```python
from build123d import *

# Parameters (mm, degrees)
SKETCH1_R           = 6.625
BOSS_EXTRUDE1_DEPTH = 3
SKETCH2_R           = 7.6
CUT_EXTRUDE1_DEPTH  = 2
BOSS_EXTRUDE2_DEPTH = 90


with BuildPart() as part:
    # Sketch1 → Boss-Extrude1 (new body)
    with BuildSketch(Plane(origin=(0, 0, 0), x_dir=(1, 0, 0), z_dir=(0, 1, 0))):
        with BuildLine():
            Line((58, -58), (58, 58))
            ThreePointArc((58, 58), (0, 116), (-58, 58))
            Line((-58, 58), (-58, -58))
            ThreePointArc((-58, -58), (0, -116), (58, -58))
        make_face()
        with Locations((0, 106.699495206)):
            Circle(SKETCH1_R, mode=Mode.SUBTRACT)
        with Locations((42.175, 33.650252397)):
            Circle(SKETCH1_R, mode=Mode.SUBTRACT)
        with Locations((-42.175, 33.650252397)):
            Circle(SKETCH1_R, mode=Mode.SUBTRACT)
        with Locations((-42.175, -33.650252397)):
            Circle(SKETCH1_R, mode=Mode.SUBTRACT)
        with Locations((0, -106.699495206)):
            Circle(SKETCH1_R, mode=Mode.SUBTRACT)
        with Locations((42.175, -33.650252397)):
            Circle(SKETCH1_R, mode=Mode.SUBTRACT)
    extrude(amount=BOSS_EXTRUDE1_DEPTH)

    # Sketch2 → Cut-Extrude1 (cut)
    with BuildSketch(Plane.XZ):
        with Locations((42.175, -33.650252397)):
            Circle(SKETCH2_R)
        with Locations((-42.175, -33.650252397)):
            Circle(SKETCH2_R)
        with Locations((0, -106.699495206)):
            Circle(SKETCH2_R)
        with Locations((42.175, 33.650252397)):
            Circle(SKETCH2_R)
        with Locations((0, 106.699495206)):
            Circle(SKETCH2_R)
        with Locations((-42.175, 33.650252397)):
            Circle(SKETCH2_R)
    extrude(amount=-CUT_EXTRUDE1_DEPTH, mode=Mode.SUBTRACT)

    # Sketch3 → Boss-Extrude2 (add, symmetric)
    with BuildSketch(Plane.XY):
        Polygon((-23, 5), (-25, 5), (-25, 3), (-28, 3), (-28, 6), (-23, 6), align=None)
        Polygon((28, 3), (28, 6), (23, 6), (23, 5), (25, 5), (25, 3), align=None)
    extrude(amount=BOSS_EXTRUDE2_DEPTH, both=True)


solid = part.part
```
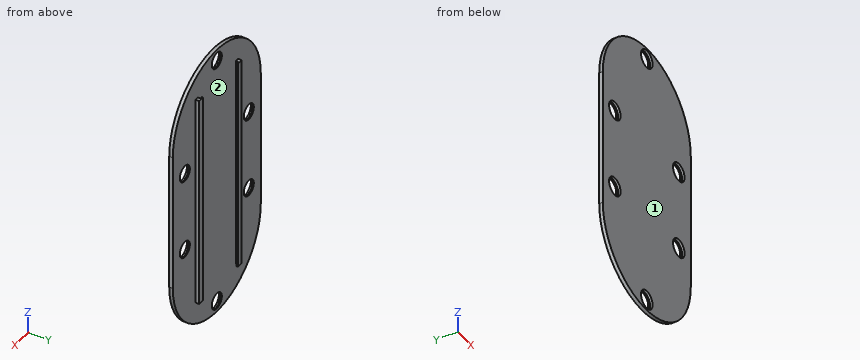
CAD build for the part. Positions are in the model's coordinates, mm. Face numbers are marked on the shaded views. Coordinates: 2 decimals unless noted, no trailing zeros. Write each loop counter-clockwise with the first axis right and the second up, starting at its lowest first coordinate (ties: lowest second). Pieces come first, ordered by that corner, then holes.
(1) Cut at A-A, the plane x = 0. List the corners of the cut face in (y, z).
(2) Two-plate mould, pull along X, no slides. Class the marked faces 1 and 2: +X half, -X half, draft (parallel to the pull), parting line (faces both ways), or undercut.
(3) Cut at B-B, the plane y = 4.1. List the corners of the cut face in (x, z), and give its area (3 significant figures).
(4) Cut at D-D, the plane x = -43. List the corners of the cut face in (y, z), and give its area (3 significant figures).
(5) Cut at C-C, the plane z = -5.5. List the corners of the cut face in (x, y).
(6) Flat gauge pins, fed straight in: pin 1 (4.5 mm diameter, centred on x = 44, z = 37, fed in from -Y); pin 2 (7.5 mm diameter, centred on x = -2, z = 104, fed in from -Y); pin 3 (1 mm diameter, centred on y = 4, z = 42.5, fed in from +X); pin 4 (0.5 mm diameter, centred on y = 5.5, z = -39, fed in from -X). Where does each tip first touch, or does it go through?
(7) Drill centre lines: probe 1 along X at (y, z) = (5.75, 51.5); probe 2 along Z at (x, y) = (0, 0.5); probe 3 along Z at (x, y) = (-42, 0.45). Where is each one in solid material? Low to high.
Geometry says:
1. outline: (0, -116) - (3, -116) - (3, -113.32) - (2, -113.32) - (2, -114.3) - (0, -114.3) - close; (0, -99.1) - (2, -99.1) - (2, -100.07) - (3, -100.07) - (3, 100.07) - (2, 100.07) - (2, 99.1) - (0, 99.1) - close; (0, 114.3) - (2, 114.3) - (2, 113.32) - (3, 113.32) - (3, 116) - (0, 116) - close
2. face 1: draft
2. face 2: undercut
3. outline: (-28, -90) - (-25, -90) - (-25, 90) - (-28, 90) - close; (25, -90) - (28, -90) - (28, 90) - (25, 90) - close
3. area: 1,080 mm2
4. outline: (0, -96.92) - (3, -96.92) - (3, -40.22) - (2, -40.22) - (2, -41.21) - (0, -41.21) - close; (0, -26.1) - (2, -26.1) - (2, -27.08) - (3, -27.08) - (3, 27.08) - (2, 27.08) - (2, 26.1) - (0, 26.1) - close; (0, 41.21) - (2, 41.21) - (2, 40.22) - (3, 40.22) - (3, 96.92) - (0, 96.92) - close
4. area: 495 mm2
5. outline: (-58, 0) - (58, 0) - (58, 3) - (28, 3) - (28, 6) - (23, 6) - (23, 5) - (25, 5) - (25, 3) - (-25, 3) - (-25, 5) - (-23, 5) - (-23, 6) - (-28, 6) - (-28, 3) - (-58, 3) - close
6. pin 1: passes through
6. pin 2: stops at y = 2
6. pin 3: stops at x = 28
6. pin 4: stops at x = -28
7. probe 1: x = -28 to -23, 23 to 28
7. probe 2: z = -116 to -114.3, -99.1 to 99.1, 114.3 to 116
7. probe 3: z = -98 to -41.25, -26.05 to 26.05, 41.25 to 98
